```python
from build123d import *

# Parameters (mm, degrees)
F2_SIZE = 0.508
F3_R    = 2.54


with BuildPart() as f1:
    # F0 (on Front) → F1 (revolve)
    with BuildSketch(Plane.XZ):
        Polygon((0, 5.55625), (0, 4), (6.35, 4), (6.35, 0), (12.7, 0), (12.7, 9.525), (0, 9.525), (0, 7.14375), (1.397, 7.14375), (1.397, 5.55625), align=None)
    revolve(axis=Axis((9.525, 0, 0), (-1, 0, 0)))

    # F2
    f2_edges = [f1.edges().sort_by_distance(p)[0] for p in [
        (0, 0, -4),
    ]]
    chamfer(f2_edges, length=F2_SIZE)

    # F3
    f3_edges = [f1.edges().sort_by_distance(p)[0] for p in [
        (12.7, 0, -9.525),
    ]]
    fillet(f3_edges, radius=F3_R)


solid = f1.part
```
Geometry check sheet. Reference: the model listing, model coordinates, mm. A direction names the side the tool comes from. Round coordinates to 2 decimals unless told otherwise and drop trailing zeros. Order: outer loops, then holes, each group sorted by start corner. A loop starts at its lowest first (then second) coordinate and runs counter-clockwise, first axis right, second up. Notation, with made-up numbers: (-29.5, 78) - (26.5, 78) arc R30 cw to (26.5, 117) - close; hole circle Ø11 at (-19, -19). An arc over 180 degrees is marked (long way). Use a Markdown table: item, result. Add a question column.
1) Section check A-A (y = 0). Record the cut outline in (x, z) (3 decimals), then the cut area to 3 significant figures.
2) Gauge pin test, flat ends, axial feed: P1, Ø5, axis at x = 6, z = -6, coming from the -Y side; P2, Ø4, axis at y = 1, z = 0, coming from the -X side; P3, Ø4, axis at x = 1.5, z = 2.5, coming from the -Y side. Record the tip position at first contact, or that the pin passes through.
3) Section check D-D (x = 9.5). Record the cut outline in (y, z) (3 decimals), then the cut area to 3 significant figures.
4) Mould release check, pull along Y, two halves, no side actions. Record for faces 3 (the cylindrical face through (0.708, 0.314, -7.137)), 4 (the flat face through (0, 5, 0)), 5 (the flat face through (6.35, 0, 0)), 6 (the cylindrical face through (5.009, -5.796, -7.559)): released by +Y, released by -Y, zero draft, split by the parting line, or undercut.
5) Thickness scan on line 1 along Y through (x, z) = (0.8, 0) (3 decimals); line 2 along Y through (x, z) = (4.15, 0) (3 decimals); line 3 along X through (y, z) = (-5.75, -3.75). Record the ranges inside material, lowest first.
6) Set-up check for faces 1 (the flat face through (1.397, -6, 0)), 2 (the flat face through (0, 6.4, 3.5)): record each of +Z, -Z, +X, -X, +Y, -Y from which the full face is reachable in a straight line by a thin tool's end or side.
7) Section check C-C (x = 4.25). Record the cut outline in (y, z) (3 decimals), then the cut area to 3 significant figures.
Established:
| question | item | result |
|---|---|---|
| 1 | outline | (0, -9.525) - (10.16, -9.525) arc R2.54 ccw to (12.7, -6.985) - (12.7, 6.985) arc R2.54 ccw to (10.16, 9.525) - (0, 9.525) - (0, 7.144) - (1.397, 7.144) - (1.397, 5.556) - (0, 5.556) - (0, 4.508) - (0.508, 4) - (6.35, 4) - (6.35, -4) - (0.508, -4) - (0, -4.508) - (0, -5.556) - (1.397, -5.556) - (1.397, -7.144) - (0, -7.144) - close |
| 1 | area | 184 mm2 |
| 2 | P1 | y = -8.86 |
| 2 | P2 | x = 6.35 |
| 2 | P3 | y = -9.51 |
| 3 | outline | circle Ø19.05 at (0, 0) |
| 3 | area | 285 mm2 |
| 4 | face 3 | undercut |
| 4 | face 4 | zero draft |
| 4 | face 5 | undercut |
| 4 | face 6 | split by the parting line |
| 5 | line 1 | -9.525 to -7.144, -5.556 to -4, 4 to 5.556, 7.144 to 9.525 |
| 5 | line 2 | -9.525 to -4, 4 to 9.525 |
| 5 | line 3 | 1.4 to 12.7 |
| 6 | face 1 | -X |
| 6 | face 2 | +Z, -Z, -X, +Y, -Y |
| 7 | outline | circle Ø19.05 at (0, 0); hole circle Ø8 at (0, 0) |
| 7 | area | 235 mm2 |
